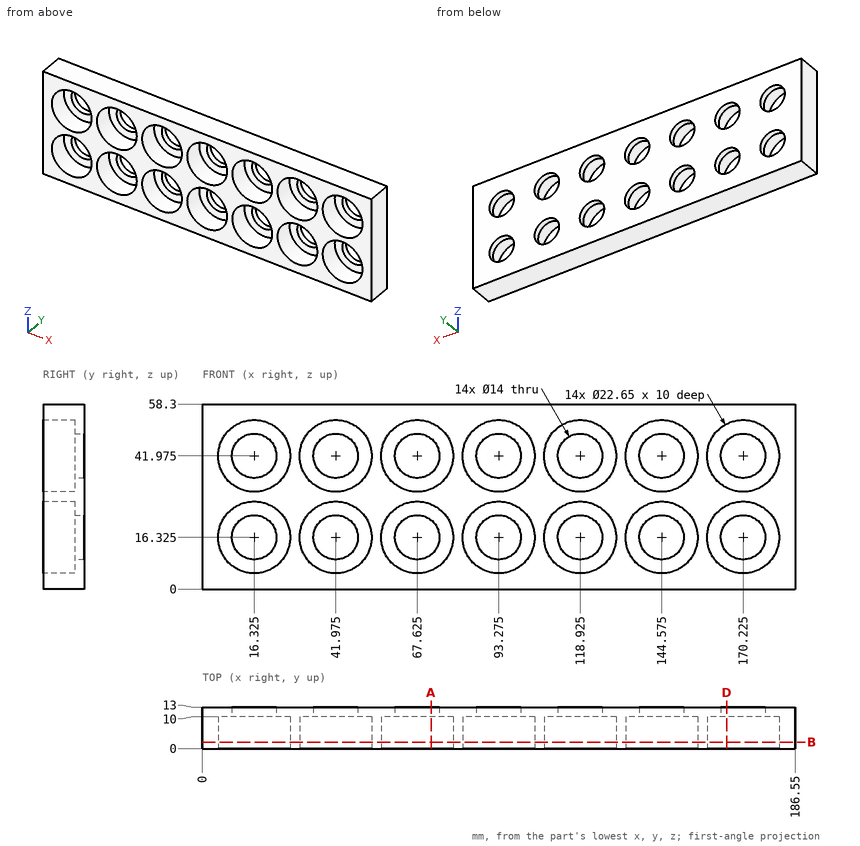
Can you work these out from the drawing? Everything is in mm from the part's minimum corner. Coordinates: 2 decimals unless noted, no trailing zeros. Loops run counter-clockwise (first coordinate to the right, second up) from the corner with the lowest first, then second, coordinate; pieces in that order, holes last.
1) Imagine slicing it at A-A on x = 72. List the corners of the cut face in (y, z) for me.
2) Imagine slicing it at B-B on y = 2. State how many separate pieces and enclosed holes the cut face has, plus the area to 3 significant figures.
3) For pin 1 (20.5 mm diameter, centred on x = 67.625, z = 16.325, fed in from -Y), with a flat end and sliding along its axis, tell me the tip position at first contact or that it passes through.
4) Imagine slicing it at D-D on x = 165. List the corners of the cut face in (y, z) for me, plus the area to 3 significant figures.
5) I need wall thicknesses on probe 1 along Z at (x, y) = (85.5, 1.5); probe 2 along Z at (x, y) = (26, 2); probe 3 along Y at (x, z) = (95, 51.5). Which ranges of each line are inside material? Lowest first, please.
Completed:
1. outline: (0, 0) - (13, 0) - (13, 10.86) - (10, 10.86) - (10, 5.88) - (0, 5.88) - close; (0, 26.77) - (10, 26.77) - (10, 21.79) - (13, 21.79) - (13, 36.51) - (10, 36.51) - (10, 31.53) - (0, 31.53) - close; (0, 52.42) - (10, 52.42) - (10, 47.44) - (13, 47.44) - (13, 58.3) - (0, 58.3) - close
2. separate pieces: 1
2. enclosed holes: 14
2. area: 5,230 mm2
3. pin 1: stops at y = 10
4. outline: (0, 0) - (13, 0) - (13, 11.67) - (10, 11.67) - (10, 6.28) - (0, 6.28) - close; (0, 26.37) - (10, 26.37) - (10, 20.98) - (13, 20.98) - (13, 37.32) - (10, 37.32) - (10, 31.93) - (0, 31.93) - close; (0, 52.02) - (10, 52.02) - (10, 46.63) - (13, 46.63) - (13, 58.3) - (0, 58.3) - close
4. area: 300 mm2
5. probe 1: z = 0 to 8.09, 24.56 to 33.74, 50.21 to 58.3
5. probe 2: z = 0 to 10.44, 22.21 to 36.09, 47.86 to 58.3
5. probe 3: y = 10 to 13
